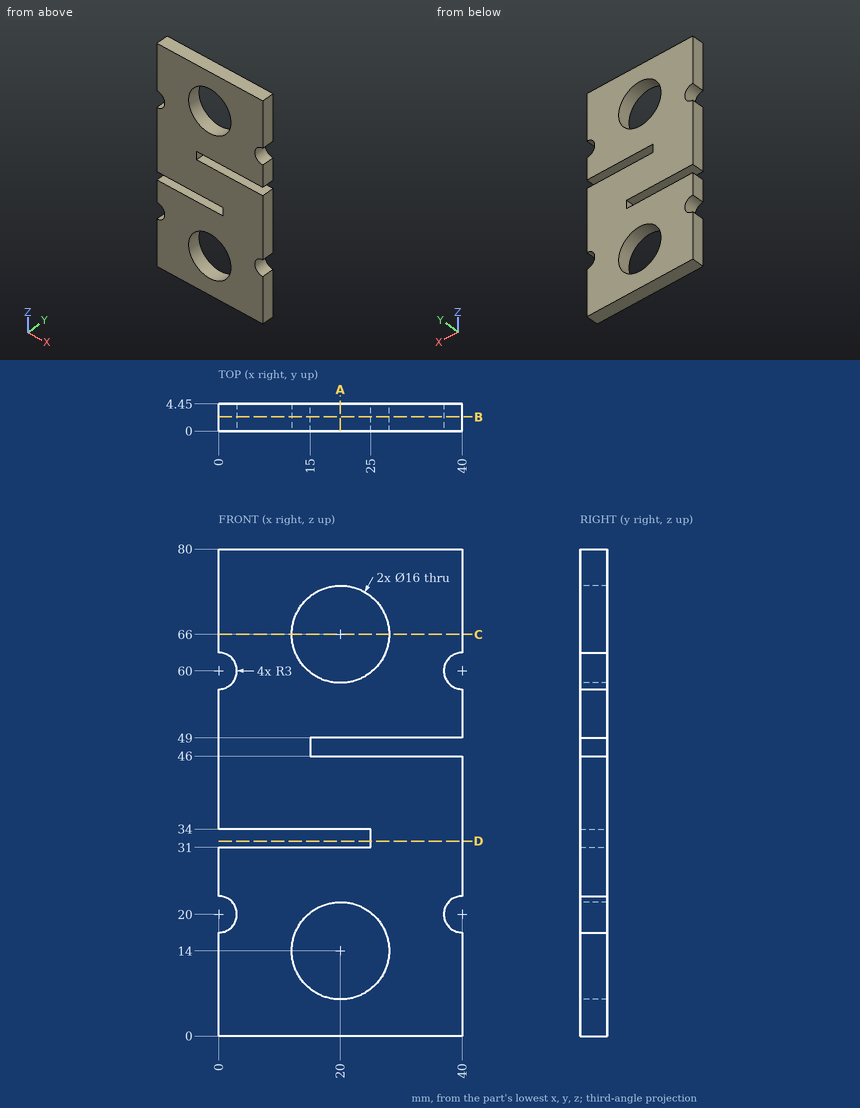
Here's the drawing with two shaded views (mm, measured from the low corner). I have some questions. Coordinates: 2 decimals unless noted, no trailing zeros. Order: outer loops, then holes, each group sorted by start corner. A loop starts at its lowest first (then second) coordinate and runs counter-clockwise, first axis right, second up.
Q1. Suppose I cut it at D-D on z = 32. Please give me the cut outline in (x, y).
Q2. Suppose I cut it at A-A on x = 20. Please give me the cut outline in (y, z), and give its area (3 significant figures).
Q3. Suppose I cut it at C-C on z = 66. Please give me the cut outline in (x, y).
Q4. Please list where these lines run through material, in increasing order: L1, parallel to Z at x = 20, y = 3.4; L2, parallel to Z at x = 6.5, y = 4; L3, parallel to Z at x = 28.5, y = 2.35.
Q5. Will this pin go through, and if not, where does the flat tip stop? pin 1 (0.9 mm diameter, centred on y = 3, z = 32.5, fed in from -X).
Q6. Suppose I cut it at B-B on y = 2.35. Please give me the cut outline in (x, z), and give its area (3 significant figures).
Answer:
1. outline: (25, 0) - (40, 0) - (40, 4.45) - (25, 4.45) - close
2. outline: (0, 0) - (4.45, 0) - (4.45, 6) - (0, 6) - close; (0, 22) - (4.45, 22) - (4.45, 31) - (0, 31) - close; (0, 34) - (4.45, 34) - (4.45, 46) - (0, 46) - close; (0, 49) - (4.45, 49) - (4.45, 58) - (0, 58) - close; (0, 74) - (4.45, 74) - (4.45, 80) - (0, 80) - close
2. area: 187 mm2
3. outline: (0, 0) - (12, 0) - (12, 4.45) - (0, 4.45) - close; (28, 0) - (40, 0) - (40, 4.45) - (28, 4.45) - close
4. L1: z = 0 to 6, 22 to 31, 34 to 46, 49 to 58, 74 to 80
4. L2: z = 0 to 31, 34 to 80
4. L3: z = 0 to 46, 49 to 80
5. pin 1: stops at x = 25
6. outline: (0, 0) - (40, 0) - (40, 17) arc R3 cw to (40, 23) - (40, 46) - (15, 46) - (15, 49) - (40, 49) - (40, 57) arc R3 cw to (40, 63) - (40, 80) - (0, 80) - (0, 63) arc R3 cw to (0, 57) - (0, 34) - (25, 34) - (25, 31) - (0, 31) - (0, 23) arc R3 cw to (0, 17) - close; hole circle Ø16 at (20, 14); hole circle Ø16 at (20, 66)
6. area: 2,590 mm2
